Here's the drawing with two shaded views (mm, measured from the low corner). I have some questions. Coordinates: 2 decimals unless noted, no trailing zeros. Write each loop counter-clockwise with the first axis right and the second up, starting at its lowest first coordinate (ties: lowest second). Pieces come first, ordered by that corner, then holes.
Item 1: If I drill on probe 1 along Y at (x, z) = (30, 8.75); probe 2 along X at (y, z) = (34, 9.25); probe 3 along X at (y, z) = (22.5, 11.5), over which ranges is the centre line in solid material (lowest first)?
Item 2: I want a section at C-C on z = 8. Please give me the cut outline in (x, y).
Item 3: I want a section at A-A on y = 30. Please give me the cut outline in (x, z).
Item 4: Thinking about a two-plate mould opening in X: for the marked faces 1, 2, 3 and 4, which applies, +X half, -X half, draft (parallel to the pull), parting line (faces both ways), or undercut?
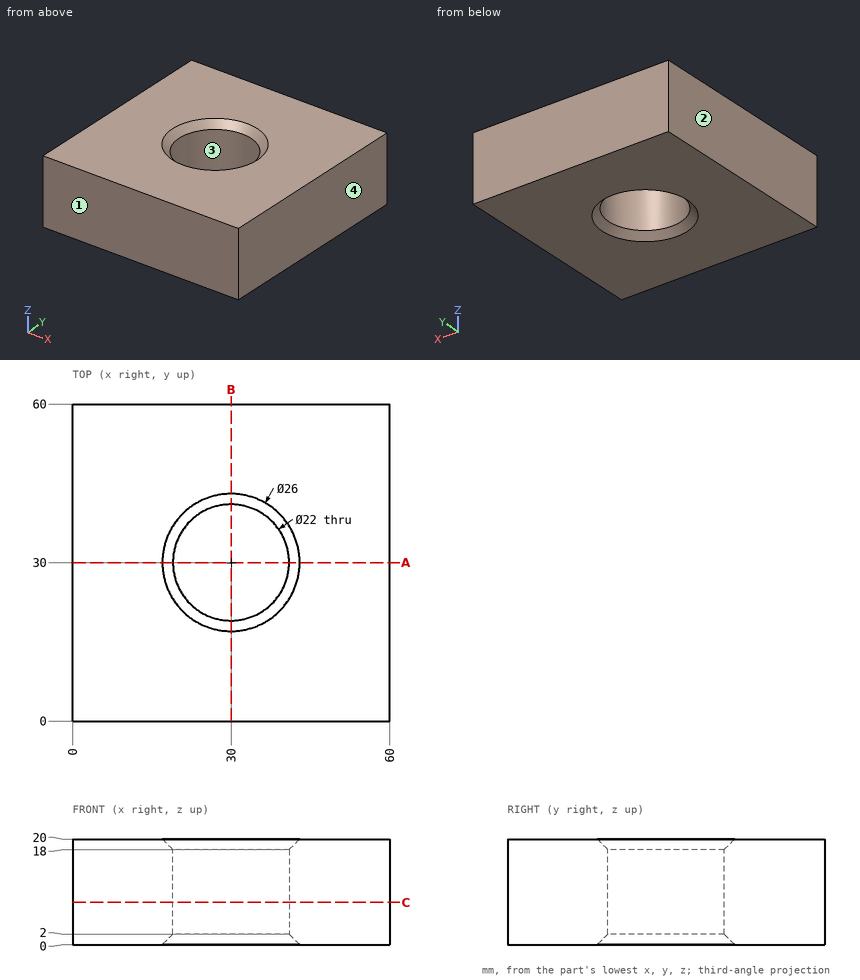
Response values:
1. probe 1: y = 0 to 19, 41 to 60
1. probe 2: x = 0 to 19.75, 40.25 to 60
1. probe 3: x = 0 to 21.95, 38.05 to 60
2. outline: (0, 0) - (60, 0) - (60, 60) - (0, 60) - close; hole circle Ø22 at (30, 30)
3. outline: (0, 0) - (17, 0) - (19, 2) - (19, 18) - (17, 20) - (0, 20) - close; (41, 2) - (43, 0) - (60, 0) - (60, 20) - (43, 20) - (41, 18) - close
4. face 1: draft
4. face 2: -X half
4. face 3: undercut
4. face 4: +X half
